from build123d import *

# Parameters (mm, degrees)
SKETCH_1_W           = 16.2
SKETCH_1_H           = 16.2
SKETCH_1_W_2         = 12.7
SKETCH_1_H_2         = 12.7
EXTRUDE_1_DEPTH      = 39
SKETCH_3_W           = 12.7
SKETCH_3_H           = 12.7
EXTRUDE_2_DEPTH      = 4
SKETCH_5_W           = 24.32
SKETCH_5_H           = 20
SKETCH_5_W_2         = 2.6
SKETCH_5_H_2         = 10.16
SKETCH_5_W_3         = 14.7
SKETCH_5_H_3         = 14.7
EXTRUDE_3_DEPTH      = 20
SKETCH_9_W           = 2.74
SKETCH_9_H           = 10.6
CUT_EXTRUDE_5_DEPTH  = 8.416671881
SKETCH_13_W          = 8.4
SKETCH_13_H          = 8.4
SKETCH_13_W_2        = 5.6
SKETCH_13_H_2        = 5.6
EXTRUDE_6_DEPTH      = 5.1
SKETCH_27_W          = 5.6
SKETCH_27_H          = 5.6
SKETCH_27_R          = 2.65
EXTRUDE_10_DEPTH     = 3.7
CUT_EXTRUDE_10_REACH = 47.485
SKETCH_33_R          = 2.65
CUT_EXTRUDE_13_REACH = 49.947
SKETCH_23_W          = 3.8
SKETCH_23_H          = 2.8
SKETCH_34_W          = 24.32
SKETCH_34_H          = 20
SKETCH_34_W_2        = 16.2
SKETCH_34_H_2        = 16.2
EXTRUDE_11_DEPTH     = 4
SKETCH_35_W          = 3
SKETCH_35_H          = 15
EXTRUDE_12_DEPTH     = 4.3
SKETCH_38_W          = 4.3
SKETCH_38_H          = 15
EXTRUDE_13_DEPTH     = 9
CUT_EXTRUDE_14_REACH = 53.972
SKETCH_39_W          = 2.94
SKETCH_39_H          = 12.6
SKETCH_23_4_W        = 13.25
SKETCH_23_4_H        = 2.74
CUT_EXTRUDE_16_DEPTH = 10
SKETCH_42_W          = 3
SKETCH_42_H          = 19.2
EXTRUDE_14_DEPTH     = 5
SKETCH_45_W          = 1.5
SKETCH_45_H          = 19.2
EXTRUDE_15_DEPTH     = 3
SKETCH_46_W          = 2.935
SKETCH_46_H          = 2.74
CUT_EXTRUDE_18_DEPTH = 10
CUT_EXTRUDE_19_REACH = 48.4
SKETCH_47_W          = 10.6
SKETCH_47_H          = 2.74
SKETCH_49_W          = 6
SKETCH_49_H          = 0.8
EXTRUDE_17_DEPTH     = 5


with BuildPart() as part:
    # Sketch 1 → Extrude 1 (new body)
    with BuildSketch(Plane(origin=(0, 0, 0), x_dir=(1, 0, 0), z_dir=(0, 1, 0))):
        Rectangle(SKETCH_1_W, SKETCH_1_H)
        Rectangle(SKETCH_1_W_2, SKETCH_1_H_2, mode=Mode.SUBTRACT)
    extrude(amount=EXTRUDE_1_DEPTH)



with BuildPart() as body_2:
    # Sketch 3 → Extrude 2 (new body)
    with BuildSketch(Plane(origin=(0, 0, 0), x_dir=(1, 0, 0), z_dir=(0, 1, 0))):
        Rectangle(SKETCH_3_W, SKETCH_3_H)
    extrude(amount=EXTRUDE_2_DEPTH)


with BuildPart() as part_1:
    add(part.part)

    add(body_2.part)  # Extrude 3 merges body 2
    # Sketch 5 → Extrude 3 (add)
    # profile 1 of 3: a face of its own
    with BuildSketch(Plane(origin=(0, 0, 0), x_dir=(1, 0, 0), z_dir=(0, 1, 0))):
        Rectangle(SKETCH_5_W, SKETCH_5_H)
        with Locations((-9.16, 0)):
            Rectangle(SKETCH_5_W_2, SKETCH_5_H_2, mode=Mode.SUBTRACT)
        Rectangle(SKETCH_5_W_3, SKETCH_5_H_3, mode=Mode.SUBTRACT)
        with Locations((9.16, 0)):
            Rectangle(SKETCH_5_W_2, SKETCH_5_H_2, mode=Mode.SUBTRACT)
    # profile 2 of 3: a face of its own
    with BuildSketch(Plane(origin=(0, 0, 0), x_dir=(1, 0, 0), z_dir=(0, 1, 0))):
        with Locations((-9.16, 0)):
            Rectangle(SKETCH_5_W_2, SKETCH_5_H_2)
    # profile 3 of 3: a face of its own
    with BuildSketch(Plane(origin=(0, 0, 0), x_dir=(1, 0, 0), z_dir=(0, 1, 0))):
        with Locations((9.16, 0)):
            Rectangle(SKETCH_5_W_2, SKETCH_5_H_2)
    extrude(amount=EXTRUDE_3_DEPTH)

    # Sketch 9 → Cut-Extrude 5 (cut)
    with BuildSketch(Plane(origin=(0, 0, 0), x_dir=(1, 0, 0), z_dir=(0, 1, 0))):
        with Locations((-8.89, 0)):
            Rectangle(SKETCH_9_W, SKETCH_9_H)
        with Locations((8.89, 0)):
            Rectangle(SKETCH_9_W, SKETCH_9_H)
    extrude(amount=CUT_EXTRUDE_5_DEPTH, mode=Mode.SUBTRACT)

    # Sketch 13 → Extrude 6 (add)
    with BuildSketch(Plane(origin=(0, 0, -10), x_dir=(-1, 0, 0), z_dir=(0, 0, -1))):
        with Locations((0, 12.6)):
            Rectangle(SKETCH_13_W, SKETCH_13_H)
        with Locations((0, 12.6)):
            Rectangle(SKETCH_13_W_2, SKETCH_13_H_2, mode=Mode.SUBTRACT)
    extrude(amount=EXTRUDE_6_DEPTH)

    # Sketch 27 → Extrude 10 (add)
    with BuildSketch(Plane(origin=(0, 0, -10), x_dir=(-1, 0, 0), z_dir=(0, 0, -1))):
        with Locations((0, 12.6)):
            Rectangle(SKETCH_27_W, SKETCH_27_H)
        with Locations((0, 12.6)):
            Circle(SKETCH_27_R, mode=Mode.SUBTRACT)
    extrude(amount=EXTRUDE_10_DEPTH)

    # Sketch 33 → Cut-Extrude 10 (cut, up to next)
    with BuildSketch(Plane(origin=(0, 0, -10), x_dir=(-1, 0, 0), z_dir=(0, 0, -1)), mode=Mode.PRIVATE) as cut_extrude_10_sk1:
        with Locations((0, 12.6)):
            Circle(SKETCH_33_R)
    cut_extrude_10_tool1 = extrude(cut_extrude_10_sk1.sketch, amount=-CUT_EXTRUDE_10_REACH, mode=Mode.PRIVATE) & part_1.part
    add(cut_extrude_10_tool1.solids().sort_by_distance((0, 12.6, -10))[0], mode=Mode.SUBTRACT)

    # Sketch 23 → Cut-Extrude 13 (cut, up to next)
    with BuildSketch(Plane.XY.offset(10), mode=Mode.PRIVATE) as cut_extrude_13_sk1:
        with Locations((0, 12.6)):
            Rectangle(SKETCH_23_W, SKETCH_23_H)
    cut_extrude_13_tool1 = extrude(cut_extrude_13_sk1.sketch, amount=-CUT_EXTRUDE_13_REACH, mode=Mode.PRIVATE) & part_1.part
    add(cut_extrude_13_tool1.solids().sort_by_distance((0, 12.6, 10))[0], mode=Mode.SUBTRACT)

    # Sketch 34 → Extrude 11 (add)
    with BuildSketch(Plane(origin=(0, 20, 0), x_dir=(1, 0, 0), z_dir=(0, 1, 0))):
        Rectangle(SKETCH_34_W, SKETCH_34_H)
        Rectangle(SKETCH_34_W_2, SKETCH_34_H_2, mode=Mode.SUBTRACT)
    extrude(amount=EXTRUDE_11_DEPTH)

    # Sketch 35 → Extrude 12 (add)
    with BuildSketch(Plane(origin=(12.16, 0, 0), x_dir=(0, 0, -1), z_dir=(1, 0, 0))):
        with Locations((8.5, 12.6)):
            Rectangle(SKETCH_35_W, SKETCH_35_H)
    extrude(amount=EXTRUDE_12_DEPTH)

    # Sketch 38 → Extrude 13 (add)
    with BuildSketch(Plane(origin=(0, 0, -10), x_dir=(-1, 0, 0), z_dir=(0, 0, -1))):
        with Locations((-14.31, 12.6)):
            Rectangle(SKETCH_38_W, SKETCH_38_H)
    extrude(amount=EXTRUDE_13_DEPTH)

    # Sketch 39 → Cut-Extrude 14 (cut, up to next)
    with BuildSketch(Plane(origin=(16.46, 0, 0), x_dir=(0, 0, -1), z_dir=(1, 0, 0)), mode=Mode.PRIVATE) as cut_extrude_14_sk1:
        with Locations((15.67, 12.6)):
            Rectangle(SKETCH_39_W, SKETCH_39_H)
    cut_extrude_14_tool1 = extrude(cut_extrude_14_sk1.sketch, amount=-CUT_EXTRUDE_14_REACH, mode=Mode.PRIVATE) & part_1.part
    add(cut_extrude_14_tool1.solids().sort_by_distance((16.46, 12.6, -15.67))[0], mode=Mode.SUBTRACT)

    # Sketch 23_4 → Cut-Extrude 16 (cut)
    with BuildSketch(Plane.XY.offset(10)):
        with Locations((0, 2.17)):
            Rectangle(SKETCH_23_4_W, SKETCH_23_4_H)
    extrude(amount=-CUT_EXTRUDE_16_DEPTH, mode=Mode.SUBTRACT)

    # Sketch 42 → Extrude 14 (add)
    with BuildSketch(Plane.XY.offset(10)):
        with Locations((-8.125, 10.4)):
            Rectangle(SKETCH_42_W, SKETCH_42_H)
    extrude(amount=EXTRUDE_14_DEPTH)

    # Sketch 45 → Extrude 15 (add)
    with BuildSketch(Plane(origin=(-6.625, 0, 0), x_dir=(0, 0, -1), z_dir=(1, 0, 0))):
        with Locations((-14.25, 10.4)):
            Rectangle(SKETCH_45_W, SKETCH_45_H)
    extrude(amount=EXTRUDE_15_DEPTH)

    # Sketch 46 → Cut-Extrude 18 (cut)
    with BuildSketch(Plane.XY.offset(10)):
        with Locations((8.0925, 2.17)):
            Rectangle(SKETCH_46_W, SKETCH_46_H)
    extrude(amount=-CUT_EXTRUDE_18_DEPTH, mode=Mode.SUBTRACT)

    # Sketch 47 → Cut-Extrude 19 (cut, up to next)
    with BuildSketch(Plane.XY, mode=Mode.PRIVATE) as cut_extrude_19_sk1:
        with Locations((-1.325, 2.17)):
            Rectangle(SKETCH_47_W, SKETCH_47_H)
    cut_extrude_19_tool1 = extrude(cut_extrude_19_sk1.sketch, amount=-CUT_EXTRUDE_19_REACH, mode=Mode.PRIVATE) & part_1.part
    add(cut_extrude_19_tool1.solids().sort_by_distance((-1.325, 2.17, 0))[0], mode=Mode.SUBTRACT)

    # Sketch 49 → Extrude 17 (add)
    with BuildSketch(Plane.XY.offset(10)):
        with Locations((-6.625, 0.4)):
            Rectangle(SKETCH_49_W, SKETCH_49_H)
    extrude(amount=EXTRUDE_17_DEPTH)


solid = part_1.part
Part model, mm, in its own coordinate system. A direction names the side the tool comes from. Round coordinates to 2 decimals unless told otherwise and drop trailing zeros. Order: outer loops, then holes, each group sorted by start corner. A loop starts at its lowest first (then second) coordinate and runs counter-clockwise, first axis right, second up. Notation, with made-up numbers: (23.5, 18.25) -> (69.5, 18.25) arc R21 ccw to (69.5, 55.25) -> close; hole circle Ø8 at (-39.75, -21). An arc over 180 degrees is marked (long way). Put each result on its own line as item: value.
Q1. Band-saw the part on D-D (z = -3). Give the cut face in (x, y) (3 decimals).
From the geometry:
outline: (-12.16, 0) -> (-10.26, 0) -> (-10.26, 8.417) -> (-7.52, 8.417) -> (-7.52, 0) -> (7.52, 0) -> (7.52, 8.417) -> (10.26, 8.417) -> (10.26, 0) -> (12.16, 0) -> (12.16, 24) -> (8.1, 24) -> (8.1, 39) -> (6.35, 39) -> (6.35, 4) -> (-6.35, 4) -> (-6.35, 39) -> (-8.1, 39) -> (-8.1, 24) -> (-12.16, 24) -> close; hole (-6.625, 0.8) -> (3.975, 0.8) -> (3.975, 3.54) -> (-6.625, 3.54) -> close
Q2. Band-saw the part on A-A (y = 7). State how many separate pieces and enclosed holes the cut face has, and give its area (3 significant figures).
From the geometry:
separate pieces: 2
enclosed holes: 3
area: 325 mm2
Q3. Band-saw the part on B-B (z = -11.5). Give the cut face in (x, y).
From the geometry:
outline: (-4.2, 8.4) -> (4.2, 8.4) -> (4.2, 16.8) -> (-4.2, 16.8) -> close; (12.16, 5.1) -> (16.46, 5.1) -> (16.46, 20.1) -> (12.16, 20.1) -> close; hole circle Ø5.3 at (0, 12.6)
Q4. Tool access for faces 4 (the face through (9, 5, 5.3)), 5 (the face through (-6.35, 21, 0)), 6 (the face through (14, 6.3, -16)), 7 (the face through (1.9, 13, 8)): list every direction of +Z, -Z, +X, -X, +Y, -Y with a clear straight run to the whole face (end or side of a thin tool).
From the geometry:
face 4: -Y
face 5: +Y
face 6: +X, -X
face 7: +Z, -Z
Q5. Wall check: line 1 (Y direction, x = -3.75, z = 7); line 2 (X direction, y = 14.5, z = -5.5); line 3 (Y direction, x = 0, z = -11.8). Give the ranges that are in metal, low to high. Write a range as [from, to].
From the geometry:
line 1: y = [0, 0.8], [3.54, 39]
line 2: x = [-12.16, -6.35], [6.35, 12.16]
line 3: y = [8.4, 9.95], [15.25, 16.8]
Q6. Pull direction Z, two halves, no side cores. Call faces 1 (the face through (14, 13, -17.14)), 2 (the face through (0, 16.8, -13)), 3 (the face through (14, 12, -7)): pulls with the +Z half, pulls with the -Z half, needs draft (parallel to the pull), parting line crosses it, or undercut.
From the geometry:
face 1: undercut
face 2: needs draft
face 3: pulls with the +Z half
Q7. Pin check, flat tips, straight feed: pin 1 Ø4 at (x, z) = (-1, 0.5) entering from +Y; pin 2 Ø3.5 at (x, z) = (15.5, -10.5) entering from +Y; pin 3 Ø1.5 at (x, y) = (10, 5) entering from -Z. Stop position of each tip, or through.
From the geometry:
pin 1: stops at y = 4
pin 2: stops at y = 20.1
pin 3: stops at z = -10
